Geometry: see drawing. Coordinates: mm, zero at the bounding-box minimum. Round coordinates to 2 decimals unless told otherwise and drop trailing zeros. Loops run counter-clockwise (first coordinate to the right, second up) from the corner with the lowest first, then second, coordinate; pieces in that order, holes last.
(1) Cut plane D-D, the plane z = 66. Output: boundary loops of the cut face in (x, y) (1 decimal), and give its area (3 significant figures).
(2) Cut plane C-C, the plane y = 2.4. Give the number of separate pieces and of enclosed holes in the cut face, and give its area (3 significant figures).
(3) Line query: line 1 (Z direction, x = 74, y = 1.5); line 2 (Z direction, x = 8, y = 1.2); line 3 (X direction, y = 1.4, z = 5.5) (1 decimal). Output: solid intervals per line, ascending.
(4) Cut plane B-B, the plane x = 75. Output: boundary loops of the cut face in (y, z) (1 decimal), and give its area (3 significant figures).
(5) Cut plane A-A, the plane x = 8. Output: boundary loops of the cut face in (y, z) (3 decimals), and give its area (3 significant figures).
(6) First-contact query: pin 1 Ø12 at (x, z) = (74.5, 33.5) entering from -Y; pin 2 Ø1.5 at (y, z) = (2, 73.5) entering from -X; pin 3 Ø1.5 at (y, z) = (2, 6) entering from -X; pin 4 Ø0.9 at (y, z) = (1.5, 5.5) entering from +X. Flat tips, straight axial feed; report the tip coordinate or a pass-through.
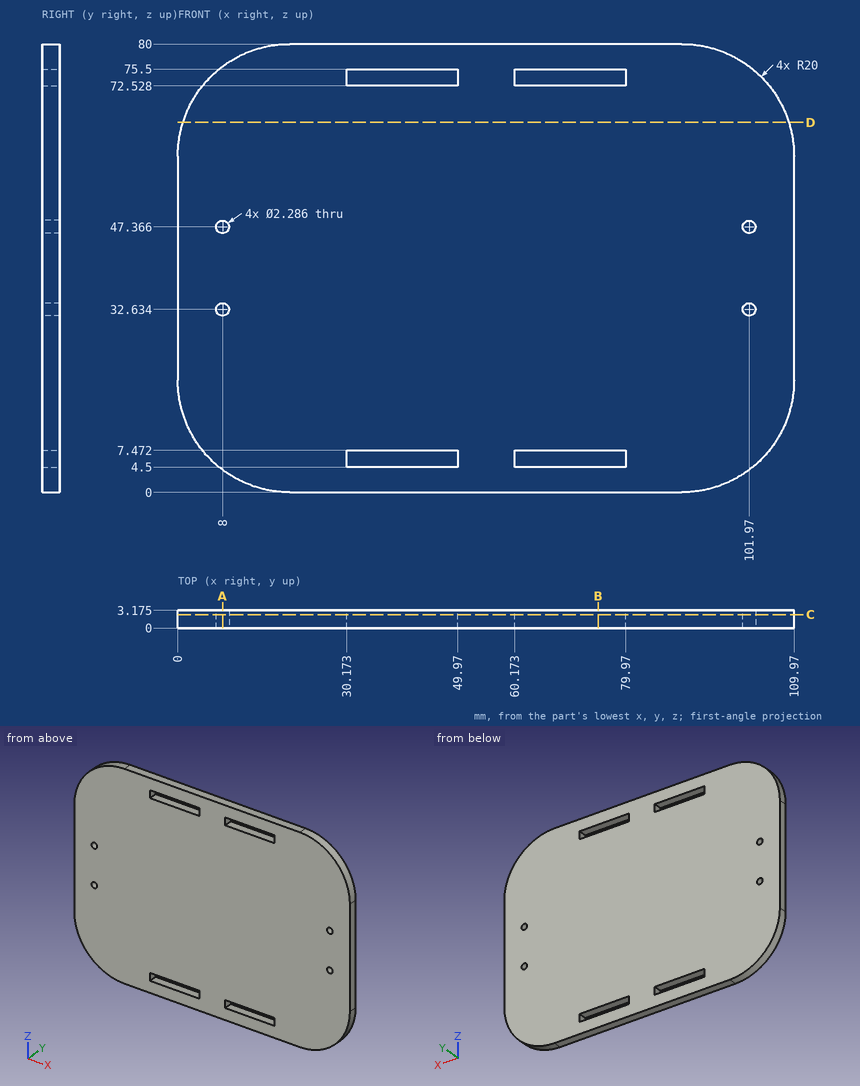
Reported:
1. outline: (0.9, 0) - (109, 0) - (109, 3.2) - (0.9, 3.2) - close
1. area: 343 mm2
2. separate pieces: 1
2. enclosed holes: 8
2. area: 8,200 mm2
3. line 1: z = 0 to 4.5, 7.47 to 72.53, 75.5 to 80
3. line 2: z = 4 to 31.49, 33.78 to 46.22, 48.51 to 76
3. line 3: x = 6.2 to 30.2, 50 to 60.2, 80 to 103.7
4. outline: (0, 0) - (3.2, 0) - (3.2, 4.5) - (0, 4.5) - close; (0, 7.5) - (3.2, 7.5) - (3.2, 72.5) - (0, 72.5) - close; (0, 75.5) - (3.2, 75.5) - (3.2, 80) - (0, 80) - close
4. area: 235 mm2
5. outline: (0, 4) - (3.175, 4) - (3.175, 31.491) - (0, 31.491) - close; (0, 33.777) - (3.175, 33.777) - (3.175, 46.223) - (0, 46.223) - close; (0, 48.509) - (3.175, 48.509) - (3.175, 76) - (0, 76) - close
5. area: 214 mm2
6. pin 1: stops at y = 0
6. pin 2: stops at x = 4.59
6. pin 3: stops at x = 5.02
6. pin 4: stops at x = 104.2
